```python
from build123d import *

# Parameters (mm, degrees)
BOSS_EXTRUDE1_DEPTH = 0.4
BOSS_EXTRUDE2_DEPTH = 3
CHAMFER1_SIZE       = 1
SKETCH4_W           = 34
SKETCH4_H           = 43
BOSS_EXTRUDE3_DEPTH = 2.5
BOSS_EXTRUDE4_DEPTH = 10
CUT_EXTRUDE1_REACH  = 7.9
SKETCH6_W           = 22
SKETCH6_H           = 6
SKETCH7_W           = 34
SKETCH7_H           = 43
BOSS_EXTRUDE5_DEPTH = 2


with BuildPart() as part:
    # Sketch2 → Boss-Extrude1 (new body)
    with BuildSketch(Plane(origin=(0, 0, 0), x_dir=(1, 0, 0), z_dir=(0, 1, 0))):
        Polygon((11, 0), (-11, 0), (-11, 6), (-15.5, 6), (-15.5, 47), (9.5, 47), (9.5, 35), (2.5, 35), (2.5, 6), (11, 6), align=None)
    extrude(amount=BOSS_EXTRUDE1_DEPTH)

    # Sketch3 → Boss-Extrude2 (add)
    with BuildSketch(Plane(origin=(0, 0.4, 0), x_dir=(1, 0, 0), z_dir=(0, 1, 0))):
        Polygon((-15.5, 6), (2.5, 6), (2.5, 35), (9.5, 35), (9.5, 47), (-15.5, 47), align=None)
    extrude(amount=BOSS_EXTRUDE2_DEPTH)

    # Chamfer1
    chamfer1_edges = [part.edges().sort_by_distance(p)[0] for p in [
        (11, 0.2, 0),
        (-11, 0.2, 0),
    ]]
    chamfer(chamfer1_edges, length=CHAMFER1_SIZE)

    # Sketch4 → Boss-Extrude3 (add)
    with BuildSketch(Plane(origin=(0, 3.4, 0), x_dir=(1, 0, 0), z_dir=(0, 1, 0))):
        with Locations((-0.5, 27.5)):
            Rectangle(SKETCH4_W, SKETCH4_H)
    extrude(amount=BOSS_EXTRUDE3_DEPTH)

    # Sketch5 → Boss-Extrude4 (add)
    with BuildSketch(Plane.XZ.offset(-3.4)):
        Polygon((-15.5, -6), (-17.5, -6), (-17.5, -49), (16.5, -49), (16.5, -6), (14.5, -6), (14.5, -47), (-15.5, -47), align=None)
    extrude(amount=BOSS_EXTRUDE4_DEPTH)

    # Sketch6 → Cut-Extrude1 (cut, up to next)
    with BuildSketch(Plane.XZ, mode=Mode.PRIVATE) as cut_extrude1_sk1:
        with Locations((0, -3)):
            Rectangle(SKETCH6_W, SKETCH6_H)
    cut_extrude1_tool1 = extrude(cut_extrude1_sk1.sketch, amount=-CUT_EXTRUDE1_REACH, mode=Mode.PRIVATE) & part.part
    add(cut_extrude1_tool1.solids().sort_by_distance((0, 0, -3))[0], mode=Mode.SUBTRACT)

    # Sketch7 → Boss-Extrude5 (add)
    with BuildSketch(Plane.XZ.offset(6.6)):
        with Locations((-0.5, -27.5)):
            Rectangle(SKETCH7_W, SKETCH7_H)
    extrude(amount=BOSS_EXTRUDE5_DEPTH)


solid = part.part
```
Verification items for the finished model (mm, model axes). A direction names the side the tool comes from. Coordinates: 2 decimals unless noted, no trailing zeros. Write each loop counter-clockwise with the first axis right and the second up, starting at its lowest first coordinate (ties: lowest second). Pieces come first, ordered by that corner, then holes. Notation, with made-up numbers: M 68.5,-10 L 75.5,-10 A19 ccw 75.5,2 Z; hole C 33.5,59 d10. An arc over 180 degrees is marked long. Answer as a JSON object with one key per item and string values. Group by question number.
(1) Material ranges on line 1 (Y direction, x = -10, z = -22); line 2 (Y direction, x = 3.5, z = -14); line 3 (X direction, y = -0.25, z = -46.5), recorded low to high.
(2) Tool access check on faces 4 (the face through (2.5, 2, -20)), 5 (the face through (-17.5, -1, -28)). Record the directions out of +Z, -Z, +X, -X, +Y, -Y that give a thin tool (end or side, any length) a straight path to the whole face; none if there is none.
(3) Cross-section at D-D, the plane z = -32.5. Record the cut outline in (x, y).
(4) Release check for a two-part mould opening along Y. For faces 1 (the face through (-1, -8.6, -27)), 2 (the face through (6, 2, -35)), 3 (the face through (-4.5, 0.4, -6)) record: +Y half, -Y half, draft (parallel to the pull), parting line (faces both ways), or undercut.
(5) Cross-section at C-C, the plane x = 1.5. Record the cut outline in (y, z).
(6) Cross-section at B-B, the plane y = -5.5. Record the cut outline in (x, z), and give its area (3 significant figures).
(7) Cross-section at A-A, the plane z = -45. Record the cut outline in (x, y).
Reply:
{
 "1": {"line 1": "-8.6 to -6.6, 0 to 5.9", "line 2": "-8.6 to -6.6, 3.4 to 5.9", "line 3": "-17.5 to -15.5, 14.5 to 16.5"},
 "2": {"face 4": "+Z", "face 5": "+Z, -Z, -X, +Y, -Y"},
 "3": {"outline": "M -17.5,-8.6 L 16.5,-8.6 L 16.5,5.9 L -17.5,5.9 Z; hole M -15.5,-6.6 L 14.5,-6.6 L 14.5,3.4 L 2.5,3.4 L 2.5,0 L -15.5,0 Z"},
 "4": {"face 1": "-Y half", "face 2": "undercut", "face 3": "draft"},
 "5": {"outline": "M -8.6,-49 L 5.9,-49 L 5.9,-6 L 0,-6 L 0,-47 L -6.6,-47 L -6.6,-6 L -8.6,-6 Z"},
 "6": {"outline": "M -17.5,-49 L 16.5,-49 L 16.5,-6 L 14.5,-6 L 14.5,-47 L -15.5,-47 L -15.5,-6 L -17.5,-6 Z", "area": "232 mm²"},
 "7": {"outline": "M -17.5,-8.6 L 16.5,-8.6 L 16.5,5.9 L -17.5,5.9 Z; hole M -15.5,-6.6 L 14.5,-6.6 L 14.5,3.4 L 9.5,3.4 L 9.5,0 L -15.5,0 Z"}
}
